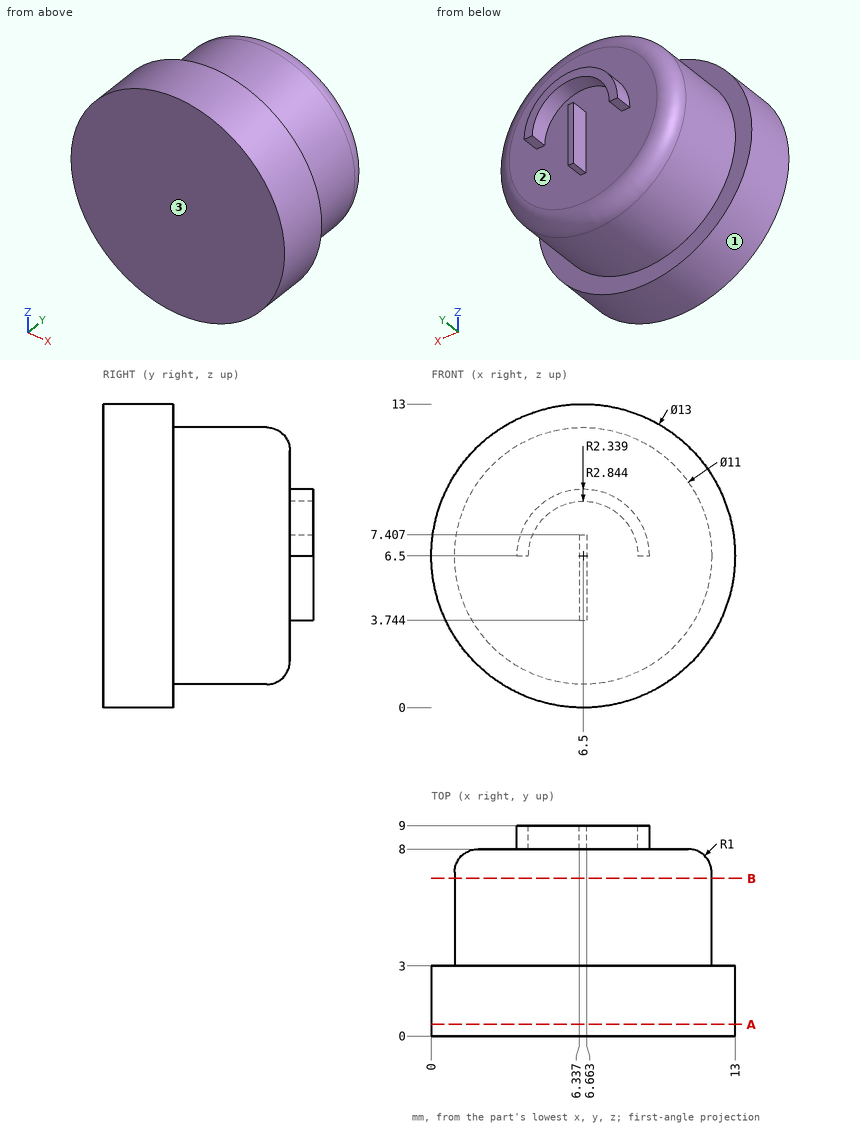
The figure shows three views and two pictorial views of one solid part (mm, origin at its lowest corner). Answer the questions. Round coordinates to 2 decimals unless told otherwise and drop trailing zeros. Loops run counter-clockwise (first coordinate to the right, second up) from the corner with the lowest first, then second, coordinate; pieces in that order, holes last. Notation, with made-up numbers: (-13.5, 47) - (13.5, 47) arc R12 cw to (13.5, 57) - close; hole circle Ø10 at (27, 64). An arc over 180 degrees is marked (long way). Use one line per item in the form item = value. Start each with the question number.
(1) Find section A-A on y = 0.5. Determine the outline of the cut face in (x, z).
(2) Flat-ended cylindrical pins translate along their axes: P1, Ø5, axis at x = 4, z = 5, coming from the -Y side; P2, Ø3, axis at y = 5.5, z = 4.5, coming from the -X side; P3, Ø0.6, axis at x = 4, y = 8.5, coming from the -Z side; P4, Ø1, axis at x = 8.5, y = 5.5, coming from the -Z side. Find the tip coordinate at first contact, or state that the pin passes through.
(3) Find section B-B on y = 6.75. Determine the outline of the cut face in (x, z).
(4) Determine the mould class of the marked faces 1, 2 and 3 for opening direction X: +X half, -X half, draft (parallel to the pull), parting line (faces both ways), or undercut.
(5) Consider line 1 (Y direction, x = 4.5, z = 10.5); line 2 (X direction, y = 7.25, z = 10.5); line 3 (Y direction, x = 1, z = 3.5). Determine where each line is inside the solid, lowest interval first.
Answer list:
q1.outline = circle Ø13 at (6.5, 6.5)
q2.P1 = 0
q2.P2 = 1.02
q2.P3 = 6.5
q2.P4 = 1.21
q3.outline = circle Ø11 at (6.5, 6.5)
q4.face_1 = parting line
q4.face_2 = undercut
q4.face_3 = draft
q5.line_1 = 0 to 8
q5.line_2 = 2.77 to 10.23
q5.line_3 = 0 to 3
